Here's how the part is built. I have some questions about the finished solid (model axes, mm). A direction names the side the tool comes from. Coordinates: 2 decimals unless noted, no trailing zeros. Write each loop counter-clockwise with the first axis right and the second up, starting at its lowest first coordinate (ties: lowest second). Pieces come first, ordered by that corner, then holes. Notation, with made-up numbers: (57.25, -19.5) -> (69.25, -19.5) arc R22 cw to (69.25, -12.5) -> close; hole circle Ø5 at (70, 55.25). An arc over 180 degrees is marked (long way). Use a Markdown table: item, result. Add a question column.
Item 1: Imagine slicing it at B-B, the plane x = 29. Write out the boundary of the cut face in (y, z), and give its area (4 significant figures).
Item 2: Will these pins go through, and if not, where does the flat tip stop? pin 1 Ø3 at (x, y) = (-1.75, 49.5) entering from +Z; pin 2 Ø4.5 at (x, y) = (-40.75, 49.5) entering from +Z; pin 3 Ø1.6 at (x, y) = (48.5, 2) entering from -Z; pin 4 Ø1 at (y, z) = (29.5, 4) entering from -X.
Item 3: Imagine slicing it at C-C, the plane z = 8.5. Write out the boundary of the cut face in (x, y).
Item 4: If I drill on line 1 along Y through (x, z) = (-51, 2); line 2 along X through (y, z) = (26.5, -11.5); line 3 along Y through (x, z) = (0, 1.85), over which ranges is the centre line in solid material (lowest first)? Write a range as from..to.
Item 5: Imagine slicing it at A-A, the plane y = 24.5. Write out the boundary of the cut face in (x, z), and give its area (3 significant figures).
Item 6: Imagine slicing it at D-D, the plane y = -8.5. Write out the boundary of the cut face in (x, z), and give its area (3 significant figures).
Item 7: If we mould it in two halves opening along Y, with no side actions, what happens to faces 6 (the conical face through (-0.376, -7.14, 30.796)), 7 (the flat face through (19, 28, 3)), 8 (the conical face through (-72.885, 12.093, 0.669))? For each: pulls with the +Y half, pulls with the -Y half, needs draft (parallel to the pull), parting line crosses it, or undercut.
Item 8: On a 3-axis mill with a long thin cutter (end or side, diameter ignored), from which of +Z, -Z, +X, -X, +Y, -Y can I reach the whole of each face in a straight line? I mean faces 1 (the flat face through (-71, 53, 0.2)), 2 (the conical face through (-72.96, 43.71, 0.67)), 3 (the flat face through (2, -11, 30)), 4 (the flat face through (114.855, 2.014, 10.086)), 5 (the flat face through (-131.1, 27.65, -16.98)). Say none if no direction works.
```python
from build123d import *

# Parameters (mm, degrees)
BOSS_EXTRUDE1_DEPTH                                  = 135
BOSS_EXTRUDE2_REACH                                  = 151.416
BOSS_EXTRUDE2_DIRECTION_2_REACH                      = 151.416
CUT_EXTRUDE1_DEPTH                                   = 50
BOSS_EXTRUDE3_DEPTH                                  = 50
SKETCH9_R                                            = 2
CUT_EXTRUDE2_DEPTH                                   = 262.164206304
CUT_EXTRUDE3_START                                   = -2
SKETCH10_W                                           = 8.681737756
SKETCH10_H                                           = 10
CUT_EXTRUDE3_DEPTH                                   = 260.164206304
SKETCH11_W                                           = 78.8
SKETCH11_H                                           = 50
SKETCH11_W_2                                         = 40.4
BOSS_EXTRUDE4_DEPTH                                  = 2
SKETCH15_W                                           = 21
SKETCH15_H                                           = 2.5
CUT_EXTRUDE8_DEPTH                                   = 2
SKETCH16_R                                           = 1.5
CUT_EXTRUDE9_DEPTH                                   = 150.530879357
SKETCH17_R                                           = 1.5
CUT_EXTRUDE10_DEPTH                                  = 189.655270521
CSK_FOR_M4_COUNTERSUNK_RAISED_HEAD_SCREW_D           = 4.5
CSK_FOR_M4_COUNTERSUNK_RAISED_HEAD_SCREW_CSINK_D     = 9.4
CSK_FOR_M4_COUNTERSUNK_RAISED_HEAD_SCREW_CSINK_ANGLE = 90
BOSS_EXTRUDE5_DEPTH                                  = 5
CUT_EXTRUDE11_DEPTH                                  = 148.817454991
CSK_FOR_M4_COUNTERSUNK_RAISED_HEAD_S_2_D             = 4.5
CSK_FOR_M4_COUNTERSUNK_RAISED_HEAD_S_2_CSINK_D       = 9.4
CSK_FOR_M4_COUNTERSUNK_RAISED_HEAD_S_2_CSINK_ANGLE   = 90
CSK_FOR_M3_COUNTERSUNK_RAISED_HEAD_SCREW_D           = 3.4
CSK_FOR_M3_COUNTERSUNK_RAISED_HEAD_SCREW_CSINK_D     = 6.3
CSK_FOR_M3_COUNTERSUNK_RAISED_HEAD_SCREW_CSINK_ANGLE = 90
CSK_FOR_M3_COUNTERSUNK_RAISED_HEAD_S_2_D             = 3.4
CSK_FOR_M3_COUNTERSUNK_RAISED_HEAD_S_2_CSINK_D       = 6.3
CSK_FOR_M3_COUNTERSUNK_RAISED_HEAD_S_2_CSINK_ANGLE   = 90


with BuildPart() as part:
    # Sketch1 → Boss-Extrude1 (new, symmetric)
    with BuildSketch(Plane(origin=(0, 0, 0), x_dir=(0, 0, -1), z_dir=(1, 0, 0))):
        Polygon((0, 0), (0, 53), (-3, 53), (-3, 3), (-40, 3), (-40, 0), (-40, -17), (-30, -17), (-30, -5), (-25, 0), align=None)
    extrude(amount=BOSS_EXTRUDE1_DEPTH, both=True)

    # Sketch2 → Cut-Revolve1 (revolve, cut)
    with BuildSketch(Plane(origin=(0, 0, 0), x_dir=(0, 0, -1), z_dir=(1, 0, 0))):
        Polygon((-66, 3), (-30, 3), (-39, -112), (-66, -112), align=None)
    revolve(axis=Axis((0, 3, 66), (0, -1, 0)), mode=Mode.SUBTRACT)

    # Sketch3 → Cut-Revolve2 (revolve, cut)
    with BuildSketch(Plane(origin=(75, 0, 0), x_dir=(0, 0, -1), z_dir=(1, 0, 0))):
        Polygon((-30, 3), (-66, 3), (-66, -112), (-39, -112), align=None)
    cut_revolve2 = revolve(axis=Axis((75, 3, 66), (0, -1, 0)), mode=Mode.SUBTRACT)

    # Sketch4 → Cut-Revolve3 (revolve, cut)
    with BuildSketch(Plane(origin=(150, 0, 0), x_dir=(0, 0, -1), z_dir=(1, 0, 0))):
        Polygon((-30, 3), (-66, 3), (-66, -112), (-39, -112), align=None)
    cut_revolve3 = revolve(axis=Axis((150, 3, 66), (0, -1, 0)), mode=Mode.SUBTRACT)

    # Boss-Extrude2: up to this face of the body (flat: up to its plane)
    boss_extrude2_end = Plane(part.part.faces().sort_by_distance((0, 53, 1.5))[0])
    # Sketch5 → Boss-Extrude2 (add, up to the picked face)
    with BuildSketch(Plane(origin=(0, 3, 0), x_dir=(1, 0, 0), z_dir=(0, 1, 0)), mode=Mode.PRIVATE) as boss_extrude2_sk1:
        Polygon((89.696341704, -3), (135, -3), (135, 27.780279129), (135, 31.407195461), (84.358099725, -3), align=None)
    boss_extrude2_tool1 = split(extrude(boss_extrude2_sk1.sketch, amount=BOSS_EXTRUDE2_REACH, mode=Mode.PRIVATE), bisect_by=boss_extrude2_end, keep=Keep.BOTH, mode=Mode.PRIVATE)
    boss_extrude2 = boss_extrude2_tool1.solids().sort_by(Axis((118.119367, 3, -8.469065), (0, 1, 0)))[0]
    add(boss_extrude2)

    # Boss-Extrude2 direction 2: up to this face of the body (flat: up to its plane)
    boss_extrude2_direction_2_end = Plane(part.part.faces().sort_by_distance((0, 0, 12.5))[0])
    # Sketch5 → Boss-Extrude2 direction 2 (add, up to the picked face)
    with BuildSketch(Plane(origin=(0, 3, 0), x_dir=(1, 0, 0), z_dir=(0, 1, 0)), mode=Mode.PRIVATE) as boss_extrude2_direction_2_sk1:
        Polygon((89.696341704, -3), (135, -3), (135, 27.780279129), (135, 31.407195461), (84.358099725, -3), align=None)
    boss_extrude2_direction_2_tool1 = split(extrude(boss_extrude2_direction_2_sk1.sketch, amount=-BOSS_EXTRUDE2_DIRECTION_2_REACH, mode=Mode.PRIVATE), bisect_by=boss_extrude2_direction_2_end, keep=Keep.BOTH, mode=Mode.PRIVATE)
    boss_extrude2_direction_2 = boss_extrude2_direction_2_tool1.solids().sort_by(Axis((118.119367, 3, -8.469065), (0, -1, 0)))[0]
    add(boss_extrude2_direction_2)

    # Sketch7 → Cut-Extrude1 (cut)
    with BuildSketch(Plane(origin=(0, 3, 0), x_dir=(1, 0, 0), z_dir=(0, 1, 0))):
        Polygon((89.696341704, -3), (135, 27.780279129), (135, -3), align=None)
    cut_extrude1 = extrude(amount=CUT_EXTRUDE1_DEPTH, mode=Mode.SUBTRACT)

    # Sketch8 → Boss-Extrude3 (add)
    with BuildSketch(Plane(origin=(0, 3, 0), x_dir=(1, 0, 0), z_dir=(0, 1, 0))):
        Polygon((135, 27.780279129), (127.311099154, 22.556274642), (135, 11.239439757), align=None)
    boss_extrude3 = extrude(amount=BOSS_EXTRUDE3_DEPTH)

    # Sketch9 → Cut-Extrude2 (cut, through all)
    with BuildSketch(Plane(origin=(97.588254801, 0, -66.303557715), x_dir=(0.5619827673392628, 0, 0.8271489401635621), z_dir=(-0.8271489401635621, 0, 0.5619827673392628))):
        with Locations((62.889245152, 33)):
            Circle(SKETCH9_R)
    cut_extrude2 = extrude(amount=-CUT_EXTRUDE2_DEPTH, mode=Mode.SUBTRACT)

    # Sketch10 → Cut-Extrude3 (cut, through all)
    with BuildSketch(Plane(origin=(97.588254801, 0, -66.303557715), x_dir=(0.5619827673392628, 0, 0.8271489401635621), z_dir=(-0.8271489401635621, 0, 0.5619827673392628)).offset(CUT_EXTRUDE3_START)):
        with Locations((62.23011403, 33)):
            Rectangle(SKETCH10_W, SKETCH10_H)
    cut_extrude3 = extrude(amount=-CUT_EXTRUDE3_DEPTH, mode=Mode.SUBTRACT)

    # Mirror1: Cut-Revolve2, Cut-Revolve3, Boss-Extrude2, Boss-Extrude2 direction 2, Cut-Extrude1, Boss-Extrude3, Cut-Extrude2, Cut-Extrude3 across plane
    add(cut_revolve2.mirror(Plane(origin=(0, 0, 0), x_dir=(0, 0, 1), z_dir=(1, 0, 0))), mode=Mode.SUBTRACT)
    add(cut_revolve3.mirror(Plane(origin=(0, 0, 0), x_dir=(0, 0, 1), z_dir=(1, 0, 0))), mode=Mode.SUBTRACT)
    add(boss_extrude2.mirror(Plane(origin=(0, 0, 0), x_dir=(0, 0, 1), z_dir=(1, 0, 0))))
    add(boss_extrude2_direction_2.mirror(Plane(origin=(0, 0, 0), x_dir=(0, 0, 1), z_dir=(1, 0, 0))))
    add(cut_extrude1.mirror(Plane(origin=(0, 0, 0), x_dir=(0, 0, 1), z_dir=(1, 0, 0))), mode=Mode.SUBTRACT)
    add(boss_extrude3.mirror(Plane(origin=(0, 0, 0), x_dir=(0, 0, 1), z_dir=(1, 0, 0))))
    add(cut_extrude2.mirror(Plane(origin=(0, 0, 0), x_dir=(0, 0, 1), z_dir=(1, 0, 0))), mode=Mode.SUBTRACT)
    add(cut_extrude3.mirror(Plane(origin=(0, 0, 0), x_dir=(0, 0, 1), z_dir=(1, 0, 0))), mode=Mode.SUBTRACT)

    # Sketch11 → Boss-Extrude4 (add)
    with BuildSketch(Plane.XY.offset(3)):
        with Locations((-26.5, 28)):
            Rectangle(SKETCH11_W, SKETCH11_H)
        with Locations((45.7, 28)):
            Rectangle(SKETCH11_W_2, SKETCH11_H)
    extrude(amount=BOSS_EXTRUDE4_DEPTH)

    # Sketch15 → Cut-Extrude8 (cut)
    with BuildSketch(Plane(origin=(0, 3, 0), x_dir=(1, 0, 0), z_dir=(0, 1, 0))):
        Polygon((-107.696902753, -17.971904438), (-125.067030496, -6.170266324), (-123.662073578, -4.102393974), (-106.291945834, -15.904032088), align=None)
        with Locations((-46, -26.25)):
            Rectangle(SKETCH15_W, SKETCH15_H)
        with Locations((-7, -26.25)):
            Rectangle(SKETCH15_W, SKETCH15_H)
        with Locations((46, -26.25)):
            Rectangle(SKETCH15_W, SKETCH15_H)
        Polygon((106.291945834, -15.904032088), (123.662073578, -4.102393974), (125.067030496, -6.170266324), (107.696902753, -17.971904438), align=None)
    extrude(amount=-CUT_EXTRUDE8_DEPTH, mode=Mode.SUBTRACT)

    # Sketch16 → Cut-Extrude9 (cut, through all)
    with BuildSketch(Plane.XY.offset(5)):
        with Locations((-1.75, 49.5)):
            Circle(SKETCH16_R)
        with Locations((-12.25, 49.5)):
            Circle(SKETCH16_R)
        with Locations((-40.75, 49.5)):
            Circle(SKETCH16_R)
        with Locations((-51.25, 49.5)):
            Circle(SKETCH16_R)
        with Locations((51.25, 49.5)):
            Circle(SKETCH16_R)
        with Locations((40.75, 49.5)):
            Circle(SKETCH16_R)
    extrude(amount=-CUT_EXTRUDE9_DEPTH, mode=Mode.SUBTRACT)

    # Sketch17 → Cut-Extrude10 (cut, through all)
    with BuildSketch(Plane(origin=(-29.722844353, 0, 43.747283073), x_dir=(0.8271489401635628, 0, 0.5619827673392619), z_dir=(-0.5619827673392618, 0, 0.8271489401635627))):
        with Locations((-94.73147838, 49.5)):
            Circle(SKETCH17_R)
        with Locations((-84.23147838, 49.5)):
            Circle(SKETCH17_R)
    cut_extrude10 = extrude(amount=-CUT_EXTRUDE10_DEPTH, mode=Mode.SUBTRACT)

    # Mirror2: Cut-Extrude10 across plane
    add(cut_extrude10.mirror(Plane(origin=(0, 0, 0), x_dir=(0, 0, 1), z_dir=(1, 0, 0))), mode=Mode.SUBTRACT)

    # CSK for M4 Countersunk Raised Head Screw (through all)
    with Locations(Plane.XY.offset(3)):
        with Locations((-70.696341704, 43), (-70.696341704, 13), (70.696341704, 43), (70.696341704, 13)):
            CounterSinkHole(CSK_FOR_M4_COUNTERSUNK_RAISED_HEAD_SCREW_D / 2, CSK_FOR_M4_COUNTERSUNK_RAISED_HEAD_SCREW_CSINK_D / 2, counter_sink_angle=CSK_FOR_M4_COUNTERSUNK_RAISED_HEAD_SCREW_CSINK_ANGLE)

    # Sketch23 → Boss-Extrude5 (add)
    with BuildSketch(Plane.XY.offset(5)):
        with BuildLine():
            Line((-7.5, 53), (-7.5, 55.5))
            ThreePointArc((-7.5, 55.5), (0, 63), (7.5, 55.5))
            Line((7.5, 55.5), (7.5, 53))
            Line((7.5, 53), (2.5, 53))
            Line((2.5, 53), (2.5, 55.5))
            ThreePointArc((2.5, 55.5), (0, 58), (-2.5, 55.5))
            Line((-2.5, 55.5), (-2.5, 53))
            Line((-2.5, 53), (-7.5, 53))
        make_face()
    extrude(amount=-BOSS_EXTRUDE5_DEPTH)

    # Sketch24 → Cut-Extrude11 (cut, through all)
    with BuildSketch(Plane(origin=(0, 28, 0), x_dir=(1, 0, 0), z_dir=(0, 1, 0))):
        Polygon((135, 14.798267743), (135, 21.735418576), (131.775310871, 19.544495475), align=None)
        Polygon((-135, 21.735418576), (-135, 14.798267743), (-131.775310871, 19.544495475), align=None)
    extrude(amount=CUT_EXTRUDE11_DEPTH, mode=Mode.SUBTRACT)

    # CSK for M4 Countersunk Raised Head S 2 (through all)
    with Locations(Plane.XY.offset(5)):
        with Locations((0, 43), (0, 13)):
            CounterSinkHole(CSK_FOR_M4_COUNTERSUNK_RAISED_HEAD_S_2_D / 2, CSK_FOR_M4_COUNTERSUNK_RAISED_HEAD_S_2_CSINK_D / 2, counter_sink_angle=CSK_FOR_M4_COUNTERSUNK_RAISED_HEAD_S_2_CSINK_ANGLE)

    # CSK for M3 Countersunk Raised Head Screw (through all)
    with Locations(Plane(origin=(0, 0, 0), x_dir=(-1, 0, 0), z_dir=(0, 0, -1))):
        with Locations((-51.25, 49.5), (-40.75, 49.5), (1.75, 49.5), (12.25, 49.5), (40.75, 49.5), (51.25, 49.5)):
            CounterSinkHole(CSK_FOR_M3_COUNTERSUNK_RAISED_HEAD_SCREW_D / 2, CSK_FOR_M3_COUNTERSUNK_RAISED_HEAD_SCREW_CSINK_D / 2, counter_sink_angle=CSK_FOR_M3_COUNTERSUNK_RAISED_HEAD_SCREW_CSINK_ANGLE)

    # CSK for M3 Countersunk Raised Head S 2 (through all)
    with Locations(Plane(origin=(-28.036896051, 0, 41.265836253), x_dir=(-0.8271489401635628, 0, -0.5619827673392619), z_dir=(0.5619827673392618, 0, -0.8271489401635627))):
        with Locations((84.23147838, 49.5), (94.73147838, 49.5)):
            csk_for_m3_countersunk_raised_head_s_2 = CounterSinkHole(CSK_FOR_M3_COUNTERSUNK_RAISED_HEAD_S_2_D / 2, CSK_FOR_M3_COUNTERSUNK_RAISED_HEAD_S_2_CSINK_D / 2, counter_sink_angle=CSK_FOR_M3_COUNTERSUNK_RAISED_HEAD_S_2_CSINK_ANGLE)

    # Mirror3: CSK for M3 Countersunk Raised Head S 2 across plane
    add(csk_for_m3_countersunk_raised_head_s_2.mirror(Plane(origin=(0, 0, 0), x_dir=(0, 0, 1), z_dir=(1, 0, 0))), mode=Mode.SUBTRACT)


solid = part.part
```
Ans:
| question | item | result |
|---|---|---|
| 1 | outline | (-17, 30) -> (-5, 30) -> (0, 25) -> (0, 0) -> (53, 0) -> (53, 5) -> (3, 5) -> (3, 40) -> (-17, 40) -> close |
| 1 | area | 552.5 mm^2 |
| 2 | pin 1 | passes through |
| 2 | pin 2 | stops at z = 5 |
| 2 | pin 3 | stops at z = 0 |
| 2 | pin 4 | stops at x = -65.9 |
| 3 | outline | (-135, 0) -> (135, 0) -> (135, 3) -> (121.64, 3) -> (121.64, 1) -> (117.19, 1) -> (117.19, 3) -> (-117.19, 3) -> (-117.19, 1) -> (-121.64, 1) -> (-121.64, 3) -> (-135, 3) -> close |
| 4 | line 1 | y = 0..47.82, 51.18..53 |
| 4 | line 2 | x = -135..-134.82, -111.04..-105.7, 105.7..111.04, 134.82..135 |
| 4 | line 3 | y = 0..10.75, 15.25..40.75, 45.25..53, 58..63 |
| 5 | outline | (-135, -31.41) -> (-88.77, 0) -> (88.77, 0) -> (135, -31.41) -> (135, -11.24) -> (127.31, -22.56) -> (89.7, 3) -> (65.9, 3) -> (65.9, 5) -> (25.5, 5) -> (25.5, 3) -> (12.9, 3) -> (12.9, 5) -> (-65.9, 5) -> (-65.9, 3) -> (-89.7, 3) -> (-127.31, -22.56) -> (-135, -11.24) -> close |
| 5 | area | 1,230 mm^2 |
| 6 | outline | (-135, 30) -> (135, 30) -> (135, 34.27) arc R35.1 cw to (126.42, 40) -> (98.58, 40) arc R35.1 cw to (51.42, 40) -> (23.58, 40) arc R35.1 cw to (-23.58, 40) -> (-51.42, 40) arc R35.1 cw to (-98.58, 40) -> (-126.42, 40) arc R35.1 cw to (-135, 34.27) -> close |
| 6 | area | 1,760 mm^2 |
| 7 | face 6 | pulls with the +Y half |
| 7 | face 7 | needs draft |
| 7 | face 8 | undercut |
| 8 | face 1 | +Z, -Z, -X, +Y |
| 8 | face 2 | +Z |
| 8 | face 3 | -Z, +X, -X, -Y |
| 8 | face 4 | +Y |
| 8 | face 5 | +Z, +Y |
